Here's how the part is built. I have some questions about the finished solid (model axes, mm). Face numbers are marked on the shaded views. A direction names the side the tool comes from. Coordinates: 2 decimals unless noted, no trailing zeros. Write each loop counter-clockwise with the first axis right and the second up, starting at its lowest first coordinate (ties: lowest second). Pieces come first, ordered by that corner, then holes. Notation, with made-up numbers: (76.25, 76.5) - (132.25, 76.5) arc R11 cw to (132.25, 85.5) - close; hole circle Ø7 at (46.25, 59.5). An arc over 180 degrees is marked (long way). Answer in a Markdown table with one row per item. Add a question column.
Item 1: Imagine slicing it at C-C (z = 17). Please give me the cut outline in (x, y).
Item 2: Imagine slicing it at D-D (x = 12). Please give me the cut outline in (y, z).
Item 3: Imagine slicing it at A-A (x = 0). Please give me the cut outline in (y, z), plus the area to 3 significant figures.
Item 4: If I drill on probe 1 along X at (y, z) = (-26.5, 22); probe 2 along Z at (x, y) = (-7, -19.5); probe 3 along Y at (x, z) = (0, 0.95), over which ranges is the centre line in solid material (lowest first)? Write a range as from..to.
Item 5: Imagine slicing it at B-B (y = 0). Please give me the cut outline in (x, z), plus the area to 3 significant figures.
Item 6: We'd pull the mould along X, two halves only. Please class the marked faces 4, 5, 6 and 7: +X half, -X half, draft (parallel to the pull), parting line (faces both ways), or undercut.
Item 7: I'm going to push flat-ended pins straight in: pin 1 (8 mm diameter, centred on y = -34.5, z = 20, fed in from -X); pin 2 (6 mm diameter, centred on x = -2.5, z = 14.5, fed in from +Y); pin 3 (9 mm diameter, centred on x = -1, y = -5, fed in from +Z). Where does each tip first touch, or does it pass through?
Item 8: Which directions (+Z, -Z, +X, -X, +Y, -Y) give clear straight access to the entire face, cutting with the end or side of a thin tool? Please do the marked faces 1, 2 and 3.
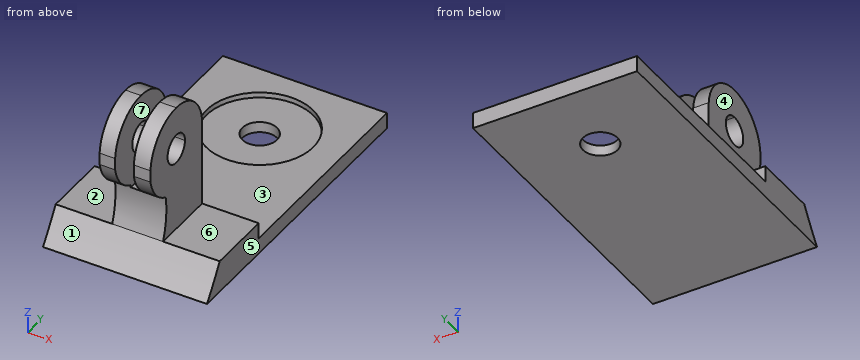
from build123d import *

# Parameters (mm, degrees)
F0_W      = 30.6736361235
F0_H      = 84.459155798
F0_R      = 3.25
F1_DEPTH  = 3
F2_W      = 30.6736361235
F2_H      = 16.2
F3_DEPTH  = 3
F4_W      = 9.5
F4_H      = 16.2
F5_DEPTH  = 24
F6_W      = 3.5
F6_H      = 16.2452395454
F7_DEPTH  = 18
F9_DEPTH  = 10
F10_R     = 10
F10_R_2   = 3.25
F11_DEPTH = 1
F12_W     = 30.6736361235
F12_H     = 28.0341655016
F13_DEPTH = 5
F15_DEPTH = 30.6746361235


# Not quite as in the source:
# - a feature names something its author has since deleted; it is built from what else it names


with BuildPart() as f1:
    # F0 (on Top) → F1 (new body)
    with BuildSketch(Plane.XY):
        Rectangle(F0_W, F0_H)
        Circle(F0_R, mode=Mode.SUBTRACT)
    extrude(amount=F1_DEPTH)

    # F2 (on face) → F3 (join)
    with BuildSketch(Plane.XY.offset(3)):
        with Locations((0, -34.129577899)):
            Rectangle(F2_W, F2_H)
    extrude(amount=F3_DEPTH)

    # F4 (on face) → F5 (join)
    with BuildSketch(Plane.XY.offset(6)):
        with Locations((0, -34.129577899)):
            Rectangle(F4_W, F4_H)
    extrude(amount=F5_DEPTH)

    # F6 (on face) → F7 (cut)
    with BuildSketch(Plane(origin=(0, -26.029577899, 0), x_dir=(-1, 0, 0), z_dir=(0, 1, 0))):
        with Locations((0.0963514363, 21.8773802273)):
            Rectangle(F6_W, F6_H)
    extrude(amount=-F7_DEPTH, mode=Mode.SUBTRACT)

    # F8 (on face) → F9 (cut)
    with BuildSketch(Plane.YZ.offset(4.75)):
        with BuildLine():
            Line((-26.029577899, 30), (-34.129577899, 30))
            Line((-34.129577899, 30), (-34.129577899, 29.9113391646))
            ThreePointArc((-34.129577899, 29.9113391646), (-28.6200020152, 27.7584969737), (-26.029577899, 22.440615928))
            Line((-26.029577899, 22.440615928), (-26.029577899, 30))
        make_face()
        with BuildLine():
            Line((-34.129577899, 29.9113391646), (-34.129577899, 30))
            Line((-34.129577899, 30), (-42.229577899, 30))
            Line((-42.229577899, 30), (-42.229577899, 22.440615928))
            ThreePointArc((-42.229577899, 22.440615928), (-39.6391537828, 27.7584969737), (-34.129577899, 29.9113391646))
        make_face()
        with BuildLine():
            ThreePointArc((-31.4004653301, 21.7848364264), (-32.1998038949, 23.7146104305), (-34.129577899, 24.5139489953))
            ThreePointArc((-34.129577899, 24.5139489953), (-36.0593519031, 19.8550624223), (-31.4004653301, 21.7848364264))
        make_face()
    extrude(amount=-F9_DEPTH, mode=Mode.SUBTRACT)

    # F10 (on face) → F11 (cut)
    with BuildSketch(Plane.XY.offset(3)):
        Circle(F10_R)
        Circle(F10_R_2, mode=Mode.SUBTRACT)
    extrude(amount=-F11_DEPTH, mode=Mode.SUBTRACT)

    # F12 (on face) → F13 (cut)
    with BuildSketch(Plane.XY.offset(3)):
        with Locations((0, 28.2124951482)):
            Rectangle(F12_W, F12_H)
    extrude(amount=-F13_DEPTH, mode=Mode.SUBTRACT)

    # F14 (on face) → F15 (cut, through all)
    with BuildSketch(Plane(origin=(-15.3368180618, 0, 0), x_dir=(0, -1, 0), z_dir=(-1, 0, 0))):
        with BuildLine():
            Line((38.2532812655, 6), (42.229577899, 6))
            Line((42.229577899, 6), (42.229577899, 20.2058496963))
            ThreePointArc((42.229577899, 20.2058496963), (40.5668907772, 16.6210972771), (37.4282303868, 14.220307964))
            ThreePointArc((37.4282303868, 14.220307964), (37.3242335364, 10.0583119864), (38.2532812655, 6))
        make_face()
        with BuildLine():
            Line((42.229577899, 0), (42.229577899, 6))
            Line((42.229577899, 6), (38.2532812655, 6))
            ThreePointArc((38.2532812655, 6), (40.1731353083, 2.9547402847), (42.229577899, 0))
        make_face()
    extrude(amount=-F15_DEPTH, mode=Mode.SUBTRACT)


solid = f1.part
Here are the results:
| question | item | result |
|---|---|---|
| 1 | outline | (-4.75, -40.85) - (-1.85, -40.85) - (-1.85, -26.03) - (-4.75, -26.03) - close; (1.65, -40.85) - (4.75, -40.85) - (4.75, -26.03) - (1.65, -26.03) - close |
| 2 | outline | (-42.23, 0) - (14.2, 0) - (14.2, 3) - (-26.03, 3) - (-26.03, 6) - (-38.25, 6) arc R79.09 cw to start |
| 3 | outline | (-42.23, 0) - (-3.25, 0) - (-3.25, 2) - (-10, 2) - (-10, 3) - (-26.03, 3) - (-26.03, 13.75) - (-37.36, 13.75) arc R16.69 cw to (-38.25, 6) arc R79.09 cw to start; (3.25, 0) - (14.2, 0) - (14.2, 3) - (10, 3) - (10, 2) - (3.25, 2) - close |
| 3 | area | 261 mm2 |
| 4 | probe 1 | x = -4.75..-1.85, 1.65..4.75 |
| 4 | probe 2 | z = 0..3 |
| 4 | probe 3 | y = -41.55..-3.25, 3.25..14.2 |
| 5 | outline | (-15.34, 0) - (-3.25, 0) - (-3.25, 2) - (-10, 2) - (-10, 3) - (-15.34, 3) - close; (3.25, 0) - (15.34, 0) - (15.34, 3) - (10, 3) - (10, 2) - (3.25, 2) - close |
| 5 | area | 59.0 mm2 |
| 6 | face 4 | -X half |
| 6 | face 5 | +X half |
| 6 | face 6 | draft |
| 6 | face 7 | undercut |
| 7 | pin 1 | stops at x = -4.75 |
| 7 | pin 2 | stops at y = -26.03 |
| 7 | pin 3 | stops at z = 2 |
| 8 | face 1 | +X, -X, -Y |
| 8 | face 2 | +Z, -X, +Y, -Y |
| 8 | face 3 | +Z, +X, -X, +Y |
